Autodesk Inventor part; units mm, degrees
ref_plane "YZ Plane" through (0, 0, 0) normal (1, 0, 0) x (0, 1, 0)
ref_plane "XZ Plane" through (0, 0, 0) normal (0, 1, 0) x (-1, 0, 0)
ref_plane "XY Plane" through (0, 0, 0) normal (0, 0, 1) x (1, 0, 0)
sketch "スケッチ1" plane through (0, 0, 0) normal (0, 0, 1) x (1, 0, 0)
  point P0 (0, 0)
sketch "スケッチ2" plane through (0, 0, 0) normal (0, 0, 1) x (1, 0, 0)
  line L0 (70, -40) -> (-70, -40)
  line L1 (-70, -40) -> (-70, 40)
  line L2 (-70, 40) -> (70, 40)
  line L3 (70, 40) -> (70, -40)
  line L4 (70, -40) -> (-70, 40) construction
  line L5 (-70, -40) -> (70, 40) construction
  circle A0 centre (-48, -19.5) radius 6.05
  circle A1 centre (48, -19.5) radius 12.55
  circle A2 centre (48, -19.5) radius 17.5
  circle A3 centre (65.5, -19.5) radius 2.05
  circle A4 centre (48, -2) radius 2.05
  circle A5 centre (30.5, -19.5) radius 2.05
  circle A6 centre (48, -37) radius 2.05
  circle A7 centre (-48, -19.5) radius 9
  circle A8 centre (-57, -19.5) radius 1.6
  circle A9 centre (-48, -28.5) radius 1.6
  circle A10 centre (-39, -19.5) radius 1.6
  circle A11 centre (-48, -10.5) radius 1.6
  line L6 (65, 35) -> (-65, 35)
  line L7 (-65, 35) -> (-65, -35)
  line L8 (-65, -35) -> (65, -35)
  line L9 (65, -35) -> (65, 35)
  line L10 (-65, 35) -> (-65, 35) construction
  line L11 (-66.6, 35) -> (-66.6, 35)
  line L12 (-63.4, 35) -> (-63.4, 35)
  arc A12 (-63.4, 35) -> (-66.6, 35) centre (-65, 35) ccw
  arc A13 (-66.6, 35) -> (-63.4, 35) centre (-65, 35) ccw
  line L13 (-65, 35) -> (-65, 35) construction
  line L14 (-65, -35) -> (-65, -35) construction
  line L15 (-63.4, -35) -> (-63.4, -35)
  line L16 (-66.6, -35) -> (-66.6, -35)
  arc A14 (-66.6, -35) -> (-63.4, -35) centre (-65, -35) ccw
  arc A15 (-63.4, -35) -> (-66.6, -35) centre (-65, -35) ccw
  line L17 (-65, -35) -> (-65, -35) construction
  line L18 (65, 35) -> (65, 35) construction
  line L19 (63.4, 35) -> (63.4, 35)
  line L20 (66.6, 35) -> (66.6, 35)
  arc A16 (66.6, 35) -> (63.4, 35) centre (65, 35) ccw
  arc A17 (63.4, 35) -> (66.6, 35) centre (65, 35) ccw
  line L21 (65, 35) -> (65, 35) construction
  line L22 (65, -35) -> (65, -35) construction
  line L23 (66.6, -35) -> (66.6, -35)
  line L24 (63.4, -35) -> (63.4, -35)
  arc A18 (63.4, -35) -> (66.6, -35) centre (65, -35) ccw
  arc A19 (66.6, -35) -> (63.4, -35) centre (65, -35) ccw
  line L25 (65, -35) -> (65, -35) construction
  line L26 (-70, -19.5) -> (70, -19.5)
  circle A20 centre (0, -19.5) radius 9
  circle A21 centre (0, -19.5) radius 39
  line L27 (-85, 40) -> (85, 40)
  line L28 (85, 40) -> (85, 35)
  line L29 (85, 35) -> (-85, 35)
  line L30 (-85, 35) -> (-85, 40)
  line L31 (-85, 35) -> (0, 0)
  line L32 (0, 0) -> (85, 35)
  line L33 (-70, 0) -> (70, 0)
  line L34 (70, 0) -> (70, -50)
  line L35 (70, -50) -> (-70, -50)
  line L36 (-70, -50) -> (-70, 0)
  point P0 (-65, -35)
  point P1 (65, 35)
  point P2 (65, -35)
  point P3 (-39.1422, -21.0937)
  point P4 (-39.1422, -17.9063)
  point P5 (0, 40)
  point P6 (85, 40)
  point P7 (48.45, -35)
  point P8 (47.55, -35)
  point P9 (-70, 28.8235)
  point P10 (70, 28.8235)
  dimension "d9" = 35
  dimension "d15" = 18
  dimension "d0" = 140
  dimension "d1" = 80
  dimension "d5" = 12.1
  dimension "d6" = 25.1
  dimension "d10" = 4.1
  dimension "d13" = 360
  dimension "d16" = 3.2
  dimension "d19" = 360
  dimension "d21" = 5
  dimension "d22" = 0
  dimension "d23" = 90
  dimension "d24" = 3.2
  dimension "d25" = 0
  dimension "d26" = 90
  dimension "d27" = 3.2
  dimension "d28" = 0
  dimension "d29" = 90
  dimension "d30" = 3.2
  dimension "d31" = 0
  dimension "d32" = 90
  dimension "d33" = 3.2
  dimension "d36" = 20.5
  dimension "d37" = 18
  dimension "d38" = 78
  dimension "d39" = 48
  dimension "d40" = 48
  dimension "d43" = 170
  dimension "d44" = 85
  dimension "d46" = 50
extrude "押し出し1" add sketch "スケッチ2" along normal blind 3 contours L0 A21 L8 A2 A6 A18 A19 L9 A3 L26 L3 | L0 A21 L8 | L26 A3 A2 L9 L33 L3 | L0 L1 L26 L7 A15 A14 L8 A21 | A21 A2 L8 | L8 A21 A10 L26 A20 A5 A2 | L33 L9 L32 L3 | L26 A2 A3 | A3 A2 L26 | L8 A15 L7 L26 A8 A7 A9 A10 A21 | L8 A6 A2 | A2 A21 A1 L26 A3 L9 L8 A6 | A2 A5 L26 A1 A21 | L32 L9 A17 L29 L3 | L33 A4 A21 L32 L9 | L9 A2 A4 L33 | A3 L9 A2 | A2 L26 L9 A3 | A3 L9 L26 A2 | A2 L9 A3 | L1 L33 L7 L26 | A21 L26 A10 | A10 A7 A21 | A6 L8 A2 | A2 A6 | A6 L8 | A5 L26 A2 | A2 L26 A5 | L29 A16 L6 A12 L1 L2 L3 | L32 A21 L31 L7 A13 L6 A17 L9 | L9 A3 L26 A1 A21 A2 A4 | L33 A4 | A4 A2 L33 | L9 L26 A3 | L9 A19 L8 A2 | A3 L26 L9 | L1 L31 L7 L33 | L7 L33 A21 A10 A7 A11 A8 L26 | A10 L26 A7 | A7 A9 A8 L26 A0 A10 | L26 A21 A10 | A10 A21 L33 A2 A5 L26 A20 | L26 A10 A7 | A7 A10 A21 | A6 L8 A2 | L26 A5 A2 | A2 A5 L26 | A5 A2 A21 A1 L26 | L32 L31 A21 | A21 L33 L32 | A4 A2 | A4 A2 A21 L33 | L1 L29 A13 L7 L31 | L7 L31 A21 L33 | L26 A7 A8 | A8 A7 L26 | A9 A7 | A7 A9 | L26 A0 A8 A7 A11 A10 | L31 L33 A21 | A8 L26 A7 | A7 L26 A8 | L26 A0 | A0 L26 | A11 A7 | A7 A11
equation "\"d27\" = d24"
equation "\"d30\" = d24"
equation "\"d33\" = d24"
equation "\"d40\" = d39"
properties part number "aaa_small_plate_middle"
Could you check a few things on this model? Use its own coordinates, in mm. Round coordinates to 2 decimals unless told otherwise and drop trailing zeros. Order: outer loops, then holes, each group sorted by start corner. A loop starts at its lowest first (then second) coordinate and runs counter-clockwise, first axis right, second up. Notation, with made-up numbers: M 1,83.5 L 19,83.5 A10 cw 19,91.5 Z; hole C -19.5,-17.5 d9. An arc over 180 degrees is marked long. One line per item, written item: value.
(1) Imagine slicing it at B-B (y = -35). Write out the boundary of the cut face in (x, z).
Ans:
outline: M -70,0 L -66.6,0 L -66.6,3 L -70,3 Z; M -63.4,0 L 63.4,0 L 63.4,3 L -63.4,3 Z; M 66.6,0 L 70,0 L 70,3 L 66.6,3 Z
(2) Imagine slicing it at D-D (x = 48). Write out the boundary of the cut face in (y, z).
Ans:
outline: M -40,0 L -32.05,0 L -32.05,3 L -40,3 Z; M -6.95,0 L 40,0 L 40,3 L -6.95,3 Z
(3) Imagine slicing it at C-C (z = 2.15). Write out the boundary of the cut face in (x, y), and give its area (3 significant figures).
Ans:
outline: M -70,-40 L 70,-40 L 70,40 L -70,40 Z; hole C -65,-35 d3.2; hole C -65,35 d3.2; hole C 0,-19.5 d18; hole C 48,-19.5 d25.1; hole C 65,-35 d3.2; hole C 65,35 d3.2
area: 10,400 mm^2
(4) I need wall thicknesses on line 1 along X through (y, z) = (35, 2.05); line 2 along Y through (x, z) = (-65, 2.35); line 3 along X through (y, z) = (-19.5, 1.3). Which ranges of each line are inside material? Lowest first, please. Write a range as from..to.
Ans:
line 1: x = -70..-66.6, -63.4..63.4, 66.6..70
line 2: y = -40..-36.6, -33.4..33.4, 36.6..40
line 3: x = -70..-9, 9..35.45, 60.55..70
(5) If we mould it in two halves opening along Y, with no side actions, what happens to faces 1 (the flat face through (1, -40, 1)), 2 (the flat face through (-1, 1, 3)), 3 (the cylindrical face through (-63.52, -34.39, 1.48))? For each: released by +Y, released by -Y, zero draft, split by the parting line, or undercut.
Ans:
face 1: released by -Y
face 2: zero draft
face 3: undercut
(6) I'm going to push a flat-ended pin straight in: P1, Ø1.9, axis at x = -65, y = 35, coming from the +Z side. Where does the tip first touch, or does it pass through?
Ans:
P1: passes through
(7) Imagine slicing it at A-A (x = 0). Write out the boundary of the cut face in (y, z).
Ans:
outline: M -40,0 L -28.5,0 L -28.5,3 L -40,3 Z; M -10.5,0 L 40,0 L 40,3 L -10.5,3 Z
